from build123d import *

# Parameters (mm, degrees)
SKETCH2_W       = 6.35
SKETCH2_H       = 50.00625
LPATTERN1_COUNT = 6
LPATTERN1_PITCH = 6.477


with BuildPart() as part:
    # Sketch2 → Revolve1 (revolve)
    with BuildSketch(Plane.XY):
        with Locations((28.575, 25.003125)):
            Rectangle(SKETCH2_W, SKETCH2_H)
    revolve(axis=Axis((0, -40.656569806, 0), (0, 1, 0)))

    # Sketch3 → Cut-Revolve1 (revolve, cut)
    with BuildSketch(Plane.XY):
        Polygon((31.75, 46.83125), (31.369, 43.59275), (31.75, 40.35425), align=None)
    cut_revolve1 = revolve(axis=Axis((0, -40.656569806, 0), (0, 1, 0)), mode=Mode.SUBTRACT)

    # LPattern1: Cut-Revolve1 ×6
    with Locations(*[(0, -i * LPATTERN1_PITCH, 0) for i in range(1, LPATTERN1_COUNT)]):
        add(cut_revolve1, mode=Mode.SUBTRACT)


solid = part.part
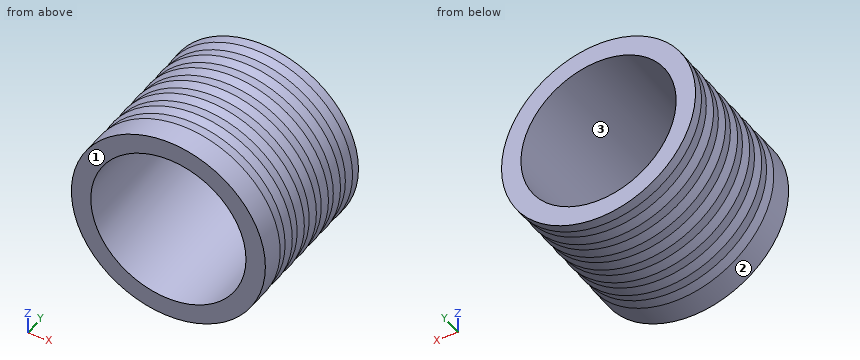
Work out the finished part from the listing and answer in its coordinate system (mm). Face numbers are marked on the shaded views. Give positions to 0.01 mm unless a question says otherwise; leave off trailing zeros. Loops run counter-clockwise (first coordinate to the right, second up) from the corner with the lowest first, then second, coordinate; pieces in that order, holes last. Notation, with made-up numbers: (-27, 60) -> (17, 60) arc R6 ccw to (17, 65) -> close; hole circle Ø5 at (33, 5). An arc over 180 degrees is marked (long way). Use a Markdown table: item, result. Add a question column.
1. Find the intervals of material crossed by probe 1 along X at (y, z) = (2.5, 5.5); probe 2 along X at (y, z) = (46, 7.5); probe 3 along Z at (x, y) = (-13, 17.5), in increasing order.
2. Section D-D on y = 29 is taken. Determine the outline of the cut face in (x, z), and give its area (3 significant figures).
3. Flat-ended cylindrical pins translate along their axes: pin 1 Ø1.5 at (x, y) = (-5, 25) entering from +Z; pin 2 Ø3 at (y, z) = (18, -3) entering from -X; pin 3 Ø10 at (y, z) = (12, -7.5) entering from -X. Find the tip coordinate at first contact, or state that the pin passes through.
4. Section C-C on y = 5 is taken. Determine the outline of the cut face in (x, z).
5. Determine the mould class of the marked faces 1, 2 and 3 for opening direction X: released by +X, released by -X, zero draft, split by the parting line, or undercut.
Results below:
| question | item | result |
|---|---|---|
| 1 | probe 1 | x = -31.27 to -24.8, 24.8 to 31.27 |
| 1 | probe 2 | x = -30.75 to -24.27, 24.27 to 30.75 |
| 1 | probe 3 | z = -28.57 to -21.82, 21.82 to 28.57 |
| 2 | outline | circle Ø63.12 at (0, 0); hole circle Ø50.8 at (0, 0) |
| 2 | area | 1,100 mm^2 |
| 3 | pin 1 | stops at z = 31.21 |
| 3 | pin 2 | stops at x = -31.48 |
| 3 | pin 3 | stops at x = -31.59 |
| 4 | outline | circle Ø63.5 at (0, 0); hole circle Ø50.8 at (0, 0) |
| 5 | face 1 | zero draft |
| 5 | face 2 | split by the parting line |
| 5 | face 3 | undercut |
